Input: part model. Units: mm. Frame: model coordinates. Coordinates: 2 decimals unless noted, no trailing zeros. Order: outer loops, then holes, each group sorted by start corner. A loop starts at its lowest first (then second) coordinate and runs counter-clockwise, first axis right, second up. Notation, with made-up numbers: M 74,58.25 L 99,58.25 A20 cw 99,69.25 Z; hole C 21,70.5 d7. An arc over 180 degrees is marked long. One line per item, written item: value.
```python
from build123d import *

# Parameters (mm, degrees)
SKETCH1_W                = 86
SKETCH1_H                = 23
EXTRUDE1_DEPTH           = 0.254
F_9_0_9_DIAMETER_HOLE1_D = 9


with BuildPart() as part:
    # Sketch1 → Extrude1 (new body)
    with BuildSketch(Plane(origin=(0, 0, 0), x_dir=(1, 0, 0), z_dir=(0, 1, 0))):
        with Locations((43, 11.5)):
            Rectangle(SKETCH1_W, SKETCH1_H)
    extrude(amount=EXTRUDE1_DEPTH)

    # Ø9.0 (9) Diameter Hole1 (through all)
    with Locations(Plane(origin=(0, 0.254, 0), x_dir=(-1, 0, 0), z_dir=(0, 1, 0))):
        with Locations((-9, -11.5), (-77, -11.5)):
            Hole(F_9_0_9_DIAMETER_HOLE1_D / 2)


solid = part.part
```
(1) Cut plane C-C on y = 0.2. Output: boundary loops of the cut face in (x, z).
Data:
outline: M 0,-23 L 86,-23 L 86,0 L 0,0 Z; hole C 9,-11.5 d9; hole C 77,-11.5 d9
(2) First-contact query: pin 1 (4 mm diameter, centred on x = 35.5, z = -11, fed in from -Y). Flat tip, straight axial feed; report the tip coordinate or a pass-through.
Data:
pin 1: stops at y = 0
(3) Cut plane B-B on z = -11.5. Output: boundary loops of the cut face in (x, y), plus the area to 3 significant figures.
Data:
outline: M 0,0 L 4.5,0 L 4.5,0.25 L 0,0.25 Z; M 13.5,0 L 72.5,0 L 72.5,0.25 L 13.5,0.25 Z; M 81.5,0 L 86,0 L 86,0.25 L 81.5,0.25 Z
area: 17.3 mm2
(4) Ray query, line 1 (X direction, y = 0.2, z = -13.25); line 2 (Z direction, x = 9, y = 0.15); line 3 (X direction, y = 0.05, z = -8.75). Return the intervals inside material, ascending. Write a range as from..to.
Data:
line 1: x = 0..4.85, 13.15..72.85, 81.15..86
line 2: z = -23..-16, -7..0
line 3: x = 0..5.44, 12.56..73.44, 80.56..86
(5) Cut plane A-A on x = 77. Output: boundary loops of the cut face in (y, z), plus the area to 3 significant figures.
Data:
outline: M 0,-23 L 0.25,-23 L 0.25,-16 L 0,-16 Z; M 0,-7 L 0.25,-7 L 0.25,0 L 0,0 Z
area: 3.56 mm2
